Can you work these out from the model? Positions are in its coordinate system, mm. Give positions to 0.01 mm unless a question says otherwise; leave off trailing zeros. Order: outer loops, then holes, each group sorted by start corner. A loop starts at its lowest first (then second) coordinate and runs counter-clockwise, first axis right, second up. Notation, with made-up numbers: (73, 0) - (112, 0) arc R28 cw to (112, 36) - close; hole circle Ø5 at (-6, -25). An arc over 180 degrees is marked (long way). Answer as a JSON object with one key per item and string values.
```python
from build123d import *

# Parameters (mm, degrees)
BOSS_EXTRUDE1_DEPTH = 3.048


with BuildPart() as part:
    # Sketch1 → Boss-Extrude1 (new body)
    with BuildSketch(Plane(origin=(0, 0, 0), x_dir=(1, 0, 0), z_dir=(0, 1, 0))):
        Polygon((-25.7556, -28.448), (-25.7556, -30.48), (-14.0716, -30.48), (-14.0716, -28.448), (13.3604, -28.448), (13.3604, -30.48), (25.0444, -30.48), (25.0444, -28.448), (43.18, -28.448), (43.18, -8.509), (27.94, -8.509), (27.94, 5.6388), (43.18, 5.6388), (43.18, 28.448), (25.0444, 28.448), (25.0444, 30.48), (13.3604, 30.48), (13.3604, 28.448), (-14.0716, 28.448), (-14.0716, 30.48), (-25.7556, 30.48), (-25.7556, 28.448), (-43.18, 28.448), (-43.18, -28.448), align=None)
    extrude(amount=BOSS_EXTRUDE1_DEPTH)


solid = part.part
```
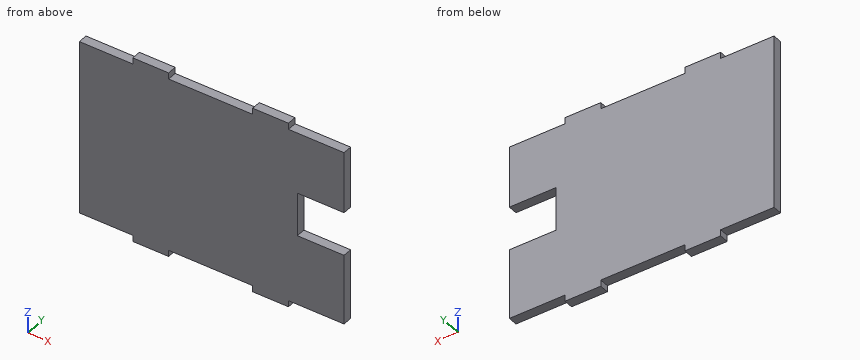
Q1. If we section it at B-B, the plane y = 2.15: Please give me the cut outline in (x, z).
Recorded:
{"outline": "(-43.18, -28.45) - (-25.76, -28.45) - (-25.76, -30.48) - (-14.07, -30.48) - (-14.07, -28.45) - (13.36, -28.45) - (13.36, -30.48) - (25.04, -30.48) - (25.04, -28.45) - (43.18, -28.45) - (43.18, -5.64) - (27.94, -5.64) - (27.94, 8.51) - (43.18, 8.51) - (43.18, 28.45) - (25.04, 28.45) - (25.04, 30.48) - (13.36, 30.48) - (13.36, 28.45) - (-14.07, 28.45) - (-14.07, 30.48) - (-25.76, 30.48) - (-25.76, 28.45) - (-43.18, 28.45) - close"}
Q2. I need wall thicknesses on L1, parallel to Z at x = 29.5, y = 1.8; L2, parallel to Z at x = -30.5, y = 2; L3, parallel to X at y = 2.25, z = 1. Which ranges of each line are inside material? Lowest first, please.
Recorded:
{"L1": "z = -28.45 to -5.64, 8.51 to 28.45", "L2": "z = -28.45 to 28.45", "L3": "x = -43.18 to 27.94"}
Q3. If we section it at D-D, the plane x = -31: Please give me the cut outline in (y, z).
Recorded:
{"outline": "(0, -28.45) - (3.05, -28.45) - (3.05, 28.45) - (0, 28.45) - close"}
Q4. I'm going to push flat-ended pins straight in: pin 1 Ø1.5 at (y, z) = (1.5, 1) entering from +X; pin 2 Ø4 at (x, z) = (0, 5) entering from -Y; pin 3 Ø0.6 at (y, z) = (1.5, 29) entering from +X; pin 4 Ø1.6 at (y, z) = (2, 30) entering from -X. Where does each tip first touch, or does it pass through?
Recorded:
{"pin 1": "stops at x = 27.94", "pin 2": "stops at y = 0", "pin 3": "stops at x = 25.04", "pin 4": "stops at x = -25.76"}
Q5. If we section it at C-C, the plane z = 1.5: Please give me the cut outline in (x, y), then the cut area to 3 significant figures.
Recorded:
{"outline": "(-43.18, 0) - (27.94, 0) - (27.94, 3.05) - (-43.18, 3.05) - close", "area": "217 mm^2"}
Q6. If we section it at A-A, the plane x = 33.5: Please give me the cut outline in (y, z).
Recorded:
{"outline": "(0, -28.45) - (3.05, -28.45) - (3.05, -5.64) - (0, -5.64) - close; (0, 8.51) - (3.05, 8.51) - (3.05, 28.45) - (0, 28.45) - close"}
